Autodesk Inventor part; units mm, degrees
ref_plane "YZ Plane" through (0, 0, 0) normal (1, 0, 0) x (0, 1, 0)
ref_plane "XZ Plane" through (0, 0, 0) normal (0, 1, 0) x (-1, 0, 0)
ref_plane "XY Plane" through (0, 0, 0) normal (0, 0, 1) x (1, 0, 0)
sketch "Sketch1" plane through (0, 0, 0) normal (0, 0, 1) x (1, 0, 0)
  line L0 (0, 0) -> (0, 8)
  line L1 (0, 8) -> (5, 8)
  line L2 (5, 8) -> (5, 6)
  line L3 (5, 6) -> (10, 6)
  line L4 (10, 6) -> (10, 8)
  line L5 (10, 8) -> (18, 8)
  line L6 (18, 8) -> (18, 0)
  line L7 (18, 0) -> (0, 0)
  dimension "d0" = 18
  dimension "d1" = 5
  dimension "d2" = 5
  dimension "d3" = 2
  dimension "d4" = 8
revolve "Revolution1" add sketch "Sketch1" angle 360 about axis through (18, 0, 0) along (-1, 0, 0)
sketch "Sketch2" plane through (0, 0, 0) normal (-1, 0, 0) x (0, 0, 1)
  circle A0 centre (0, 0) radius 8
hole "Hole1" at (0, 0, 0) direction (1, 0, 0) diameter 3 end through all countersink diameter 5 countersink angle 60
sketch "Sketch3" plane through (18, 0, 0) normal (1, 0, 0) x (0, 0, -1)
  circle A0 centre (0, 0) radius 1.5
  circle A1 centre (0, 0) radius 8
  circle A2 centre (0, 0) radius 2.5
  dimension "d13" = 5
extrude "Extrusion1" add sketch "Sketch3" along normal blind 38 contours A2
properties part number "hotend_mount" material "Aluminum 6061"
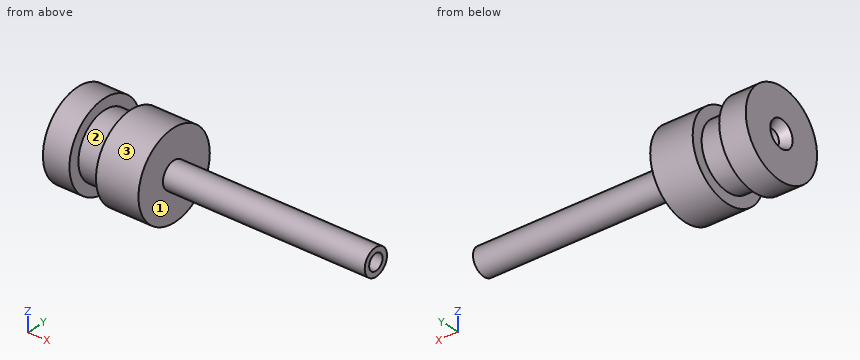
CAD build for the part. Positions are in the model's coordinates, mm. Face numbers are marked on the shaded views. A direction names the side the tool comes from. Coordinates: 2 decimals unless noted, no trailing zeros. Order: outer loops, then holes, each group sorted by start corner. A loop starts at its lowest first (then second) coordinate and runs counter-clockwise, first axis right, second up.
Item 1: Band-saw the part on A-A on y = 0. List the corners of the cut face in (x, z).
Check sheet entries:
outline: (0, -8) - (5, -8) - (5, -6) - (10, -6) - (10, -8) - (18, -8) - (18, -2.5) - (56, -2.5) - (56, -1.5) - (1.73, -1.5) - (0, -2.5) - close; (0, 2.5) - (1.73, 1.5) - (56, 1.5) - (56, 2.5) - (18, 2.5) - (18, 8) - (10, 8) - (10, 6) - (5, 6) - (5, 8) - (0, 8) - close
Item 2: 3-axis set-ups, long thin cutter, end or side, ignore diameter. For the marked faces 1, 2 and 3: which of +Z, -Z, +X, -X, +Y, -Y reach the whole face in a straight line?
Check sheet entries:
face 1: +X
face 2: none
face 3: +X, -X
Item 3: Band-saw the part on C-C on x = 6. List the corners of the cut face in (y, z), plus the area to 3 significant figures.
Check sheet entries:
outline: circle Ø12 at (0, 0); hole circle Ø3 at (0, 0)
area: 106 mm2
Item 4: Drill centre lines: L1, parallel to Z at x = 7, y = 0; L2, parallel to X at y = -5.75, z = -2.5; L3, parallel to Y at x = 11.25, z = 0. Where is each one in solid material? Low to high.
Check sheet entries:
L1: z = -6 to -1.5, 1.5 to 6
L2: x = 0 to 5, 10 to 18
L3: y = -8 to -1.5, 1.5 to 8
Item 5: Pin check, flat tips, straight feed: pin 1 Ø1 at (x, z) = (26, 0.5) entering from +Y; pin 2 Ø4 at (x, y) = (23.5, -2.5) entering from +Z; pin 3 Ø2 at (x, y) = (46.5, -3) entering from +Z. Stop position of each tip, or through.
Check sheet entries:
pin 1: stops at y = 2.5
pin 2: stops at z = 2.45
pin 3: stops at z = 1.5
Item 6: Band-saw the part on D-D on y = 6.5. List the corners of the cut face in (x, z), plus the area to 3 significant figures.
Check sheet entries:
outline: (0, -4.66) - (5, -4.66) - (5, 4.66) - (0, 4.66) - close; (10, -4.66) - (18, -4.66) - (18, 4.66) - (10, 4.66) - close
area: 121 mm2
